Could you check a few things on this model? Use its own coordinates, in mm. Coordinates: 2 decimals unless noted, no trailing zeros. Loops run counter-clockwise (first coordinate to the right, second up) from the corner with the lowest first, then second, coordinate; pieces in that order, holes last. Notation, with made-up numbers: M 62.5,19 L 114.5,19 A27 ccw 114.5,43 Z; hole C 40,78.25 d1. An arc over 180 degrees is marked long. Write each question's results on one line, items separated by ' | '.
```python
from build123d import *

# Parameters (mm, degrees)
EXTRUDE1_DEPTH      = 4
EXTRUDE2_DEPTH      = 12.357816692
EXTRUDE2_DEPTH_BACK = 12.357816692
SKETCH2_R           = 1
EXTRUDE3_DEPTH      = 12.357816692
EXTRUDE3_DEPTH_BACK = 12.357816692
SKETCH4_W           = 6
SKETCH4_H           = 8.732029078
FILLET2_R           = 1
EXTRUDE4_DEPTH      = 14
EXTRUDE4_DEPTH_BACK = 3
SKETCH3_R           = 1.5
EXTRUDE5_DEPTH      = 9
SKETCH6_R           = 1.5
EXTRUDE6_DEPTH      = 1
SKETCH7_R           = 0.6
EXTRUDE7_DEPTH      = 1
FILLET3_R           = 1
SKETCH8_R           = 2
EXTRUDE8_DEPTH      = 1
SKETCH9_R           = 15.158662045
EXTRUDE9_DEPTH      = 18.811513131
SKETCH_2_R          = 0.75
CUT_EXTRUDE_1_DEPTH = 10.447221814
FILLET_1_R          = 1


with BuildPart() as part:
    # Sketch1 → Extrude1 (new, symmetric)
    with BuildSketch(Plane.XY):
        Polygon((0, 0), (-7, 0), (-7, 8), (7, 8), (7, 0), align=None)
    extrude(amount=EXTRUDE1_DEPTH, both=True)

    # Sketch2 → Extrude2 (cut, two sides: drawn at the far end of the back side and taken through both)
    with BuildSketch(Plane.XY.offset(-EXTRUDE2_DEPTH_BACK)):
        with Locations((4.5, 5.5)):
            Circle(SKETCH2_R)
    extrude(amount=EXTRUDE2_DEPTH + EXTRUDE2_DEPTH_BACK, mode=Mode.SUBTRACT)

    # Sketch4 → Extrude3 (cut, two sides: drawn at the far end of the back side and taken through both)
    with BuildSketch(Plane(origin=(0, 0, 0), x_dir=(0, 0, -1), z_dir=(1, 0, 0)).offset(-EXTRUDE3_DEPTH_BACK)):
        with Locations((0, 5.366014539)):
            Rectangle(SKETCH4_W, SKETCH4_H)
    extrude(amount=EXTRUDE3_DEPTH + EXTRUDE3_DEPTH_BACK, mode=Mode.SUBTRACT)

    # Fillet2
    fillet2_edges = [part.edges().sort_by_distance(p)[0] for p in [
        (-7, 8, -3.5),
        (7, 8, -3.5),
        (-7, 8, 3.5),
        (7, 8, 3.5),
    ]]
    fillet(fillet2_edges, radius=FILLET2_R)

    # Sketch3 → Extrude4 (add, two sides: drawn at the far end of the back side and taken through both)
    with BuildSketch(Plane.XY.offset(-EXTRUDE4_DEPTH_BACK)):
        with Locations((-3, 4.5)):
            Circle(SKETCH3_R)
    extrude(amount=EXTRUDE4_DEPTH + EXTRUDE4_DEPTH_BACK)

    # Sketch5 → Extrude5 (cut)
    with BuildSketch(Plane.XY.offset(14)):
        Polygon((-4, 4.5), (-4, 6.060686456), (-4.95644391, 6.060686456), (-4.95644391, 2.5), (-4, 2.5), align=None)
    extrude(amount=-EXTRUDE5_DEPTH, mode=Mode.SUBTRACT)

    # Sketch6 → Extrude6 (add)
    with BuildSketch(Plane.XZ):
        with Locations((-7, 0)):
            Circle(SKETCH6_R)
        with Locations((7, 0)):
            Circle(SKETCH6_R)
    extrude(amount=-EXTRUDE6_DEPTH)

    # Sketch7 → Extrude7 (cut)
    with BuildSketch(Plane.XZ):
        with Locations((-7, 0)):
            Circle(SKETCH7_R)
        with Locations((7, 0)):
            Circle(SKETCH7_R)
    extrude(amount=-EXTRUDE7_DEPTH, mode=Mode.SUBTRACT)

    # Fillet3
    fillet3_edges = [part.edges().sort_by_distance(p)[0] for p in [
        (7, 0.5, -1.5),
        (7, 0.5, 1.5),
        (-7, 0.5, 1.5),
        (-7, 0.5, -1.5),
    ]]
    fillet(fillet3_edges, radius=FILLET3_R)

    # Sketch8 → Extrude8 (cut)
    with BuildSketch(Plane.XZ):
        Circle(SKETCH8_R)
    extrude(amount=-EXTRUDE8_DEPTH, mode=Mode.SUBTRACT)

    # Sketch9 → Extrude9 (cut, through all)
    with BuildSketch(Plane(origin=(0, 1, 0), x_dir=(1, 0, 0), z_dir=(0, 1, 0))):
        Circle(SKETCH9_R)
    extrude(amount=EXTRUDE9_DEPTH, mode=Mode.SUBTRACT)

    # Эскиз2 → Вырез-Вытянуть1 (cut, through all)
    with BuildSketch(Plane(origin=(0, 1, 0), x_dir=(1, 0, 0), z_dir=(0, 1, 0))):
        with Locations(Location((-4.5, 0, 0), (0, 0, 270))):
            Circle(SKETCH_2_R)
        with Locations(Location((4.5, 0, 0), (0, 0, 270))):
            Circle(SKETCH_2_R)
    extrude(amount=-CUT_EXTRUDE_1_DEPTH, mode=Mode.SUBTRACT)

    # Скругление1
    fillet_1_edges = [part.edges().sort_by_distance(p)[0] for p in [
        (-7, 0.5, -4),
        (-7, 0.5, 4),
        (7, 0.5, -4),
        (7, 0.5, 4),
    ]]
    fillet(fillet_1_edges, radius=FILLET_1_R)


solid = part.part
```
(1) Imagine slicing it at A-A, the plane x = 0. List the corners of the cut face in (y, z) for me.
Reported:
outline: M 0,-4 L 1,-4 L 1,-2 L 0,-2 Z; M 0,2 L 1,2 L 1,4 L 0,4 Z
(2) If we mould it in two halves opening along Z, with no side actions, what happens to faces 1 (the cylindrical face through (-7.16, 0.49, -1.75)), 2 (the cylindrical face through (7.572, 0.493, 0.18)), 3 (the flat face through (-2, 0, 1))? For each: released by +Z, released by -Z, zero draft, split by the parting line, or undercut.
Reported:
face 1: released by -Z | face 2: undercut | face 3: zero draft
(3) Imagine slicing it at C-C, the plane y = 0.2. List the corners of the cut face in (x, z) for me, and give its area (3 significant figures).
Reported:
outline: M -7.6,-1.37 A1 cw -7,-2.29 L -7,-3 A1 ccw -6,-4 L 6,-4 A1 ccw 7,-3 L 7,-2.29 A1 cw 7.6,-1.37 A1.5 ccw 7.6,1.37 A1 cw 7,2.29 L 7,3 A1 ccw 6,4 L -6,4 A1 ccw -7,3 L -7,2.29 A1 cw -7.6,1.37 A1.5 ccw Z; hole C -7,0 d1.2; hole C -4.5,0 d1.5; hole C 0,0 d4; hole C 4.5,0 d1.5; hole C 7,0 d1.2 | area: 100 mm2
(4) Please list where these lines run through material, in increasing order: probe 1 along X at (y, z) = (0.7, -0.5); probe 2 along Z at (x, y) = (0, 0.25); probe 3 along X at (y, z) = (0.1, -0.25). Write a range as from..to.
Reported:
probe 1: x = -8.41..-7.33, -6.67..-5.06, -3.94..-1.94, 1.94..3.94, 5.06..6.67, 7.33..8.41 | probe 2: z = -4..-2, 2..4 | probe 3: x = -8.48..-7.55, -6.45..-5.21, -3.79..-1.98, 1.98..3.79, 5.21..6.45, 7.55..8.48
(5) Imagine slicing it at B-B, the plane z = 0. List the corners of the cut face in (x, y) for me.
Reported:
outline: M -8.5,0 L -7.6,0 L -7.6,1 L -8.5,1 Z; M -6.4,0 L -5.25,0 L -5.25,1 L -6.4,1 Z; M -3.75,0 L -2,0 L -2,1 L -3.75,1 Z; M 2,0 L 3.75,0 L 3.75,1 L 2,1 Z; M 5.25,0 L 6.4,0 L 6.4,1 L 5.25,1 Z; M 7.6,0 L 8.5,0 L 8.5,1 L 7.6,1 Z
(6) Imagine slicing it at D-D, the plane x = -4.5. List the corners of the cut face in (y, z) for me, and give its area (3 significant figures).
Reported:
outline: M 0,-4 L 1,-4 L 1,-0.75 L 0,-0.75 Z; M 0,0.75 L 1,0.75 L 1,4 L 0,4 Z | area: 6.50 mm2
